The model under review builds one solid part; all positions refer to its coordinate system, in mm. A direction names the side the tool comes from. Coordinates: 2 decimals unless noted, no trailing zeros. Order: outer loops, then holes, each group sorted by start corner. A loop starts at its lowest first (then second) coordinate and runs counter-clockwise, first axis right, second up. Notation, with made-up numbers: M -22,18.25 L 1,18.25 A18 cw 1,41.25 Z; hole C -29,71.5 d5. An arc over 180 degrees is marked long. One line per item, written item: value.
Autodesk Inventor part; units mm, degrees
ref_plane "YZ Plane" through (0, 0, 0) normal (1, 0, 0) x (0, 1, 0)
ref_plane "XZ Plane" through (0, 0, 0) normal (0, 1, 0) x (-1, 0, 0)
ref_plane "XY Plane" through (0, 0, 0) normal (0, 0, 1) x (1, 0, 0)
sketch "Sketch1" plane through (0, 0, 0) normal (0, 0, 1) x (1, 0, 0)
  line L0 (0, 0) -> (0, 7.5)
  line L1 (0, 7.5) -> (2.4, 7.5)
  line L2 (2.4, 7.5) -> (2.4, 3)
  line L3 (2.4, 3) -> (2.9, 3)
  line L4 (2.9, 2) -> (2.4, 2) construction
  line L5 (2.4, 2) -> (2.4, 0)
  line L6 (2.4, 0) -> (0, 0)
  line L7 (2.4, 2) -> (2.9, 2.5)
  line L8 (2.9, 3) -> (2.9, 2.5)
  line L9 (2.9, 2.5) -> (2.9, 2) construction
  dimension "d0" = 2.4
  dimension "d1" = 2
  dimension "d2" = 1
  dimension "d3" = 4.5
  dimension "d7" = 45
  dimension "d8" = 0.5
revolve "Revolution1" add sketch "Sketch1" angle 360 about axis through (0, 0, 0) along (0, 1, 0)
properties part number "Stepper Shaft Extension"
(1) Insertion check: pin 1 Ø3 at (x, z) = (2, 0) entering from -Y; pin 2 Ø1.5 at (x, z) = (-2, -2.5) entering from -Y. Each pin has a flat end and moves straight along its axis. Give the tip position at first contact, or say it passes through.
Geometry results:
pin 1: stops at y = 0
pin 2: stops at y = 2.05
(2) We need section A-A, the plane x = 0. State the section outline as (y, z) points.
Geometry results:
outline: M 0,-2.4 L 2,-2.4 L 2.5,-2.9 L 3,-2.9 L 3,-2.4 L 7.5,-2.4 L 7.5,2.4 L 3,2.4 L 3,2.9 L 2.5,2.9 L 2,2.4 L 0,2.4 Z
(3) Tool access review of faces 1 (the flat face through (0, 7.5, 0)), 2 (the cylindrical face through (1.29, 5.219, 2.024)), 3 (the cylindrical face through (1.29, 0.986, 2.024)): name each direction out of +Z, -Z, +X, -X, +Y, -Y from which nothing blocks a thin tool from reaching the whole face with its end or side.
Geometry results:
face 1: +Z, -Z, +X, -X, +Y
face 2: +Y
face 3: -Y
(4) We need section B-B, the plane z = 0. State the section outline as (x, y) points.
Geometry results:
outline: M -2.9,2.5 L -2.4,2 L -2.4,0 L 2.4,0 L 2.4,2 L 2.9,2.5 L 2.9,3 L 2.4,3 L 2.4,7.5 L -2.4,7.5 L -2.4,3 L -2.9,3 Z
(5) For L1, parallel to Z at x = -0.05, y = 6.25; L2, parallel to Z at x = -1.3, y = 0.5, list the stretches that pass through material, from the lowest coordinate up.
Geometry results:
L1: z = -2.4 to 2.4
L2: z = -2.02 to 2.02
(6) We need section C-C, the plane y = 1. State the section outline as (x, z) points, plus the area to 3 significant figures.
Geometry results:
outline: C 0,0 d4.8
area: 18.1 mm2
